Check sheet for the modelled part. Datum: model origin and axes. Units: mm. A direction names the side the tool comes from. Round coordinates to 2 decimals unless told otherwise and drop trailing zeros. Write each loop counter-clockwise with the first axis right and the second up, starting at its lowest first coordinate (ties: lowest second). Pieces come first, ordered by that corner, then holes.
Item 1: Cross-section at B-B on y = 7.25. Enter the section's corners in (x, z).
Item 2: Cross-section at A-A on x = 0. Enter the section's corners in (y, z), plus the area to 3 significant figures.
Item 3: Cross-section at C-C on x = 8.5. Enter the section's corners in (y, z), plus the area to 3 significant figures.
Item 4: Cross-section at D-D on z = 4.75. Enter the section's corners in (x, y), plus the area to 3 significant figures.
Item 5: Go/stop test with flat-tipped pins: pin 1 Ø2.5 at (x, y) = (0.5, -9) entering from +Z; pin 2 Ø1.5 at (y, z) = (-5, 2) entering from -X; pin 3 Ø1.9 at (x, y) = (-8, 0) entering from +Z; pin 4 Ø2 at (y, z) = (6.5, 2.5) entering from +X. Record where each tip stops, or that it passes through.
Item 6: Release check for a two-part mould opening along X. For faces 6 (the flat face through (4.9, 0, 5)), 7 (the flat face through (0, 4.9, 5)), 8 (the cylindrical face through (-6.8, 0.05, 0.69)) record: +X half, -X half, draft (parallel to the pull), parting line (faces both ways), or undercut.
Item 7: Material ranges on line 1 (Y direction, x = 0, z = 2.7); line 2 (Y direction, x = 0, z = 0.7); line 3 (Z direction, x = 5.75, y = 1.5), recorded low to high.
Item 8: Tool access check on faces 1 (the flat face through (0, 0, 0)), 2 (the flat face through (-4.9, 0, 5)), 3 (the flat face through (-9, -1, 1.4)), 4 (the flat face through (0, -4.9, 5)), 5 (the cylindrical face through (9.2, 0.05, 0.69)). Record the directions out of +Z, -Z, +X, -X, +Y, -Y that give a thin tool (end or side, any length) a straight path to the whole face; none if there is none.
from build123d import *

# Parameters (mm, degrees)
SZKIC1_R                                          = 11
DODANIE_WYCI_GNI_CIE1_DEPTH                       = 3
POG_BIENIE_WALCOWE_POD_M2_RUB_Z_BEM_S_D           = 2.4
POG_BIENIE_WALCOWE_POD_M2_RUB_Z_BEM_S_CBORE_D     = 5
POG_BIENIE_WALCOWE_POD_M2_RUB_Z_BEM_S_CBORE_DEPTH = 1.6
SZKIC4_W                                          = 9.8
SZKIC4_H                                          = 9.8
DODANIE_WYCI_GNI_CIE2_DEPTH                       = 4.8
ZAOKR_GLENIE1_R                                   = 0.5


with BuildPart() as part:
    # Szkic1 → Dodanie-wyciągnięcie1 (new body)
    with BuildSketch(Plane.XY):
        Circle(SZKIC1_R)
    extrude(amount=DODANIE_WYCI_GNI_CIE1_DEPTH)

    # Pogłębienie walcowe pod M2 Śrubę z łbem stożkowym ściętym1 (through all)
    with Locations(Plane.XY.offset(3)):
        with Locations((-8, 0), (0, 8), (0, -8), (8, 0)):
            CounterBoreHole(POG_BIENIE_WALCOWE_POD_M2_RUB_Z_BEM_S_D / 2, POG_BIENIE_WALCOWE_POD_M2_RUB_Z_BEM_S_CBORE_D / 2, POG_BIENIE_WALCOWE_POD_M2_RUB_Z_BEM_S_CBORE_DEPTH)

    # Szkic4 → Dodanie-wyciągnięcie2 (add)
    with BuildSketch(Plane.XY.offset(3)):
        Rectangle(SZKIC4_W, SZKIC4_H)
    extrude(amount=DODANIE_WYCI_GNI_CIE2_DEPTH)

    # Zaokrąglenie1
    zaokr_glenie1_edges = [part.edges().sort_by_distance(p)[0] for p in [
        (4.9, -4.9, 5.4),
        (4.9, 4.9, 5.4),
        (-4.9, 4.9, 5.4),
        (-4.9, -4.9, 5.4),
    ]]
    fillet(zaokr_glenie1_edges, radius=ZAOKR_GLENIE1_R)


solid = part.part
Response values:
1. outline: (-8.27, 0) - (-0.94, 0) - (-0.94, 1.4) - (-2.38, 1.4) - (-2.38, 3) - (-8.27, 3) - close; (0.94, 0) - (8.27, 0) - (8.27, 3) - (2.38, 3) - (2.38, 1.4) - (0.94, 1.4) - close
2. outline: (-11, 0) - (-9.2, 0) - (-9.2, 1.4) - (-10.5, 1.4) - (-10.5, 3) - (-11, 3) - close; (-6.8, 0) - (6.8, 0) - (6.8, 1.4) - (5.5, 1.4) - (5.5, 3) - (4.9, 3) - (4.9, 7.8) - (-4.9, 7.8) - (-4.9, 3) - (-5.5, 3) - (-5.5, 1.4) - (-6.8, 1.4) - close; (9.2, 0) - (11, 0) - (11, 3) - (10.5, 3) - (10.5, 1.4) - (9.2, 1.4) - close
2. area: 90.3 mm2
3. outline: (-6.98, 0) - (-1.09, 0) - (-1.09, 1.4) - (-2.45, 1.4) - (-2.45, 3) - (-6.98, 3) - close; (1.09, 0) - (6.98, 0) - (6.98, 3) - (2.45, 3) - (2.45, 1.4) - (1.09, 1.4) - close
3. area: 31.0 mm2
4. outline: (-4.9, -4.4) arc R0.5 ccw to (-4.4, -4.9) - (4.4, -4.9) arc R0.5 ccw to (4.9, -4.4) - (4.9, 4.4) arc R0.5 ccw to (4.4, 4.9) - (-4.4, 4.9) arc R0.5 ccw to (-4.9, 4.4) - close
4. area: 95.8 mm2
5. pin 1: stops at z = 1.4
5. pin 2: stops at x = -10.15
5. pin 3: passes through
5. pin 4: stops at x = 9.53
6. face 6: +X half
6. face 7: draft
6. face 8: undercut
7. line 1: y = -11 to -10.5, -5.5 to 5.5, 10.5 to 11
7. line 2: y = -11 to -9.2, -6.8 to 6.8, 9.2 to 11
7. line 3: z = 0 to 3
8. face 1: -Z, +X, -X, +Y, -Y
8. face 2: +Z, -X, +Y, -Y
8. face 3: +Z
8. face 4: +Z, +X, -X, -Y
8. face 5: +Z, -Z
